Input: part model. Units: mm. Frame: model coordinates. A direction names the side the tool comes from. Coordinates: 2 decimals unless noted, no trailing zeros. Loops run counter-clockwise (first coordinate to the right, second up) from the corner with the lowest first, then second, coordinate; pieces in that order, holes last.
(1) Section A-A, the plane y = 3.25. Return loops of the section in (x, z), then the cut area to 3 significant figures.
(2) Section C-C, the plane z = -38.1. Return loops of the section in (x, y).
(3) Section D-D, the plane z = -12.7. Return loops of the section in (x, y), then the cut area to 3 significant figures.
(4) Set-up query: faces 1 (the face through (38.2, 19.05, -16.3)), 2 (the face through (25, 13, 0)). Return all of +Z, -Z, +X, -X, +Y, -Y with unobstructed straight access to the full face (end or side cutting, diameter ignored); none if empty.
(5) Mould query, pull axis X, two halves, no side actions, for faces 3 (the face through (50.8, 13, -25)), 4 (the face through (41.221, 9.392, -13.994)), 5 (the face through (0, 13, -25)), 6 (the face through (25, 0, -26)). Classes: released by +X, released by -X, zero draft, split by the parting line, or undercut.
(6) Section B-B, the plane x = 38.1. Return loops of the section in (y, z).
(7) Contact query for a flat-ended pin moving along its axis: P1, Ø11, axis at x = 12.7, z = -12.7, coming from the -Y side. Output: stop coordinate, or through.
(8) Line query: L1, parallel to Z at x = 12.7, y = 7; L2, parallel to Z at x = 12.7, y = 21.25; L3, parallel to X at y = 2.25, z = -37. Output: solid intervals per line, ascending.
```python
from build123d import *

# Parameters (mm, degrees)
SKETCH1_W                                        = 101.6
SKETCH1_H                                        = 50.8
BOSS_EXTRUDE1_DEPTH                              = 25.4
CBORE_FOR_1_4_SOCKET_HEAD_CAP_SCREW1_D           = 6.7564
CBORE_FOR_1_4_SOCKET_HEAD_CAP_SCREW1_CBORE_D     = 11.1125
CBORE_FOR_1_4_SOCKET_HEAD_CAP_SCREW1_CBORE_DEPTH = 6.35
LPATTERN1_COUNT                                  = 4
LPATTERN1_PITCH                                  = 25.4
F_1_4_CLEARANCE_HOLE1_D                          = 6.7564
LPATTERN2_COUNT                                  = 4
LPATTERN2_PITCH                                  = 25.4
SKETCH7_W                                        = 50.8
SKETCH7_H                                        = 25.4
CUT_EXTRUDE1_DEPTH                               = 50.8


with BuildPart() as part:
    # Sketch1 → Boss-Extrude1 (new body)
    with BuildSketch(Plane(origin=(0, 0, 0), x_dir=(1, 0, 0), z_dir=(0, 1, 0))):
        with Locations((50.8, 25.4)):
            Rectangle(SKETCH1_W, SKETCH1_H)
    extrude(amount=BOSS_EXTRUDE1_DEPTH)

    # CBORE for 1/4 Socket Head Cap Screw1 (through all)
    with Locations(Plane(origin=(0, 25.4, 0), x_dir=(-1, 0, 0), z_dir=(0, 1, 0))):
        with Locations((-12.7, -12.7)):
            cbore_for_1_4_socket_head_cap_screw1 = CounterBoreHole(CBORE_FOR_1_4_SOCKET_HEAD_CAP_SCREW1_D / 2, CBORE_FOR_1_4_SOCKET_HEAD_CAP_SCREW1_CBORE_D / 2, CBORE_FOR_1_4_SOCKET_HEAD_CAP_SCREW1_CBORE_DEPTH)

    # LPattern1: CBORE for 1/4 Socket Head Cap Screw1 ×4
    with Locations(*[(i * LPATTERN1_PITCH, 0, 0) for i in range(1, LPATTERN1_COUNT)]):
        add(cbore_for_1_4_socket_head_cap_screw1, mode=Mode.SUBTRACT)

    # 1/4 Clearance Hole1 (through all)
    with Locations(Plane(origin=(0, 25.4, 0), x_dir=(-1, 0, 0), z_dir=(0, 1, 0))):
        with Locations((-12.7, -38.1)):
            f_1_4_clearance_hole1 = Hole(F_1_4_CLEARANCE_HOLE1_D / 2)

    # LPattern2: 1/4 Clearance Hole1 ×4
    with Locations(*[(i * LPATTERN2_PITCH, 0, 0) for i in range(1, LPATTERN2_COUNT)]):
        add(f_1_4_clearance_hole1, mode=Mode.SUBTRACT)

    # Sketch7 → Cut-Extrude1 (cut)
    with BuildSketch(Plane(origin=(101.6, 0, 0), x_dir=(0, 0, -1), z_dir=(1, 0, 0))):
        with Locations((25.4, 12.7)):
            Rectangle(SKETCH7_W, SKETCH7_H)
    extrude(amount=-CUT_EXTRUDE1_DEPTH, mode=Mode.SUBTRACT)


solid = part.part
```
Report:
1. outline: (0, -50.8) - (50.8, -50.8) - (50.8, 0) - (0, 0) - close; hole circle Ø6.76 at (12.7, -38.1); hole circle Ø6.76 at (12.7, -12.7); hole circle Ø6.76 at (38.1, -38.1); hole circle Ø6.76 at (38.1, -12.7)
1. area: 2,440 mm2
2. outline: (0, 0) - (9.32, 0) - (9.32, 25.4) - (0, 25.4) - close; (16.08, 0) - (34.72, 0) - (34.72, 25.4) - (16.08, 25.4) - close; (41.48, 0) - (50.8, 0) - (50.8, 25.4) - (41.48, 25.4) - close
3. outline: (0, 0) - (9.32, 0) - (9.32, 19.05) - (7.14, 19.05) - (7.14, 25.4) - (0, 25.4) - close; (16.08, 0) - (34.72, 0) - (34.72, 19.05) - (32.54, 19.05) - (32.54, 25.4) - (18.26, 25.4) - (18.26, 19.05) - (16.08, 19.05) - close; (41.48, 0) - (50.8, 0) - (50.8, 25.4) - (43.66, 25.4) - (43.66, 19.05) - (41.48, 19.05) - close
3. area: 892 mm2
4. face 1: +Y
4. face 2: +Z, +X, -X, +Y, -Y
5. face 3: released by +X
5. face 4: undercut
5. face 5: released by -X
5. face 6: zero draft
6. outline: (0, -50.8) - (25.4, -50.8) - (25.4, -41.48) - (0, -41.48) - close; (0, -34.72) - (25.4, -34.72) - (25.4, -18.26) - (19.05, -18.26) - (19.05, -16.08) - (0, -16.08) - close; (0, -9.32) - (19.05, -9.32) - (19.05, -7.14) - (25.4, -7.14) - (25.4, 0) - (0, 0) - close
7. P1: stops at y = 0
8. L1: z = -50.8 to -41.48, -34.72 to -16.08, -9.32 to 0
8. L2: z = -50.8 to -41.48, -34.72 to -18.26, -7.14 to 0
8. L3: x = 0 to 9.51, 15.89 to 34.91, 41.29 to 50.8
